from build123d import *

# Parameters (mm, degrees)
SKETCH1_W                    = 76.2
SKETCH1_H                    = 50.8
SKETCH1_W_2                  = 63.5
SKETCH1_H_2                  = 42.333333334
BOSS_EXTRUDE1_DEPTH          = 63.5
TAP_DRILL_FOR_M10X1_5_TAP1_D = 8.5


with BuildPart() as part:
    # Sketch1 → Boss-Extrude1 (new body, symmetric)
    with BuildSketch(Plane(origin=(0, 0, 0), x_dir=(1, 0, 0), z_dir=(0, 1, 0))):
        Rectangle(SKETCH1_W, SKETCH1_H)
        Rectangle(SKETCH1_W_2, SKETCH1_H_2, mode=Mode.SUBTRACT)
    extrude(amount=BOSS_EXTRUDE1_DEPTH, both=True)

    # Tap Drill for M10x1.5 Tap1 (through all)
    with Locations(Plane.XY.offset(25.4)):
        with Locations((-12.7, 38.1), (12.7, 38.1)):
            Hole(TAP_DRILL_FOR_M10X1_5_TAP1_D / 2)


solid = part.part
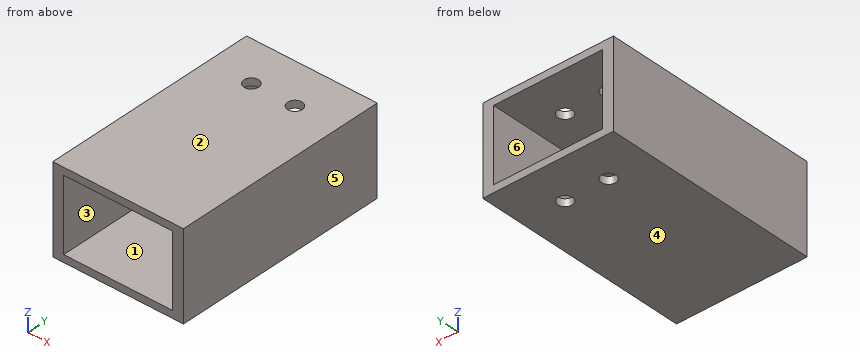
Geometry check sheet. Reference: the model listing, model coordinates, mm. Face numbers are marked on the shaded views. A direction names the side the tool comes from. Round coordinates to 2 decimals unless told otherwise and drop trailing zeros. Loops run counter-clockwise (first coordinate to the right, second up) from the corner with the lowest first, then second, coordinate; pieces in that order, holes last. Notation, with made-up numbers: (-8, 48.5) -> (19, 48.5) arc R28 cw to (19, 78.5) -> close; hole circle Ø3 at (-12.5, -30). An arc over 180 degrees is marked (long way). Answer as a JSON object with one key per item and string values. Group by question number.
Item 1: Cross-section at C-C, the plane y = 38.1. Record the cut outline in (x, z).
Item 2: Set-up check for the marked faces 1 and 2: record each of +Z, -Z, +X, -X, +Y, -Y from which the full face is reachable in a straight line by a thin tool's end or side.
Item 3: Cross-section at A-A, the plane z = 11.5. Record the cut outline in (x, y), plus the area to 3 significant figures.
Item 4: Release check for a two-part mould opening along Z. For the marked faces 3, 4, 5 and 6 record: pulls with the +Z half, pulls with the -Z half, needs draft (parallel to the pull), parting line crosses it, or undercut.
Item 5: Cross-section at D-D, the plane y = 11. Record the cut outline in (x, z).
Item 6: Thickness scan on line 1 along X through (y, z) = (38, -23); line 2 along X through (y, z) = (3.5, 4); line 3 along Z through (x, y) = (4.5, -56.5). Record the ranges inside material, lowest first.
Item 7: Depth check by flat-ended pin: pin 1 Ø5 at (x, y) = (12.7, 38.1) entering from +Z. Enter the tip coordinate at first touch or a pass-through.
Item 8: Cross-section at B-B, the plane x = 14.5. Record the cut outline in (y, z).
Determined:
{
 "1": {"outline": "(-38.1, -25.4) -> (-16.95, -25.4) -> (-16.95, -21.17) -> (-31.75, -21.17) -> (-31.75, 21.17) -> (-16.95, 21.17) -> (-16.95, 25.4) -> (-38.1, 25.4) -> close; (-8.45, -25.4) -> (8.45, -25.4) -> (8.45, -21.17) -> (-8.45, -21.17) -> close; (-8.45, 21.17) -> (8.45, 21.17) -> (8.45, 25.4) -> (-8.45, 25.4) -> close; (16.95, -25.4) -> (38.1, -25.4) -> (38.1, 25.4) -> (16.95, 25.4) -> (16.95, 21.17) -> (31.75, 21.17) -> (31.75, -21.17) -> (16.95, -21.17) -> close"},
 "2": {"face 1": "+Y, -Y", "face 2": "+Z, +X, -X, +Y, -Y"},
 "3": {"outline": "(-38.1, -63.5) -> (-31.75, -63.5) -> (-31.75, 63.5) -> (-38.1, 63.5) -> close; (31.75, -63.5) -> (38.1, -63.5) -> (38.1, 63.5) -> (31.75, 63.5) -> close", "area": "1,610 mm²"},
 "4": {"face 3": "undercut", "face 4": "pulls with the -Z half", "face 5": "needs draft", "face 6": "undercut"},
 "5": {"outline": "(-38.1, -25.4) -> (38.1, -25.4) -> (38.1, 25.4) -> (-38.1, 25.4) -> close; hole (-31.75, -21.17) -> (31.75, -21.17) -> (31.75, 21.17) -> (-31.75, 21.17) -> close"},
 "6": {"line 1": "x = -38.1 to -16.95, -8.45 to 8.45, 16.95 to 38.1", "line 2": "x = -38.1 to -31.75, 31.75 to 38.1", "line 3": "z = -25.4 to -21.17, 21.17 to 25.4"},
 "7": {"pin 1": "passes through"},
 "8": {"outline": "(-63.5, -25.4) -> (34.25, -25.4) -> (34.25, -21.17) -> (-63.5, -21.17) -> close; (-63.5, 21.17) -> (34.25, 21.17) -> (34.25, 25.4) -> (-63.5, 25.4) -> close; (41.95, -25.4) -> (63.5, -25.4) -> (63.5, -21.17) -> (41.95, -21.17) -> close; (41.95, 21.17) -> (63.5, 21.17) -> (63.5, 25.4) -> (41.95, 25.4) -> close"}
}
